```python
from build123d import *

# Parameters (mm, degrees)
SKETCH1_W           = 50
SKETCH1_H           = 100
BOSS_EXTRUDE1_DEPTH = 2.5
SKETCH2_R           = 1.25
BOSS_EXTRUDE2_DEPTH = 2.5
SKETCH4_W           = 15
SKETCH4_H           = 7.5
SKETCH4_H_2         = 33
CUT_EXTRUDE1_DEPTH  = 1


with BuildPart() as part:
    # Sketch1 → Boss-Extrude1 (new body, symmetric)
    with BuildSketch(Plane.XY):
        Rectangle(SKETCH1_W, SKETCH1_H)
    extrude(amount=BOSS_EXTRUDE1_DEPTH, both=True)

    # Sketch2 → Boss-Extrude2 (add)
    with BuildSketch(Plane.XY.offset(2.5)):
        with Locations((20, -10)):
            Circle(SKETCH2_R)
    boss_extrude2 = extrude(amount=BOSS_EXTRUDE2_DEPTH)

    # Sketch3 → Revolve1 (revolve)
    with BuildSketch(Plane(origin=(20, 0, 0), x_dir=(0, 0, -1), z_dir=(1, 0, 0))):
        with BuildLine():
            Line((-8, -6.75), (-8, -13.25))
            ThreePointArc((-8, -13.25), (-11.25, -10), (-8, -6.75))
        make_face()
    revolve1 = revolve(axis=Axis((20, -6.75, 8), (0, -1, 0)))

    # Sketch4 → Cut-Extrude1 (cut)
    with BuildSketch(Plane.XY.offset(2.5)):
        with Locations((-11.25, 37.25)):
            Rectangle(SKETCH4_W, SKETCH4_H)
        with Locations((11.25, 37.25)):
            Rectangle(SKETCH4_W, SKETCH4_H)
        with Locations((11.25, 10)):
            Rectangle(SKETCH4_W, SKETCH4_H_2)
        with Locations((-11.25, 10)):
            Rectangle(SKETCH4_W, SKETCH4_H_2)
        with Locations((-11.25, -30)):
            Rectangle(SKETCH4_W, SKETCH4_H_2)
        with Locations((11.25, -30)):
            Rectangle(SKETCH4_W, SKETCH4_H_2)
    cut_extrude1 = extrude(amount=-CUT_EXTRUDE1_DEPTH, mode=Mode.SUBTRACT)

    # Mirror1: Boss-Extrude2, Revolve1, Cut-Extrude1 across plane
    add(boss_extrude2.mirror(Plane.XY))
    add(revolve1.mirror(Plane.XY))
    add(cut_extrude1.mirror(Plane.XY), mode=Mode.SUBTRACT)


solid = part.part
```
Design review of the part built by this model. Coordinates are the model's own, in mm. A direction names the side the tool comes from. Round coordinates to 2 decimals unless told otherwise and drop trailing zeros. Write each loop counter-clockwise with the first axis right and the second up, starting at its lowest first coordinate (ties: lowest second). Pieces come first, ordered by that corner, then holes. Notation, with made-up numbers: (-14.75, -33) -> (24.25, -33) arc R31 ccw to (24.25, -2) -> close; hole circle Ø9 at (12, -40). An arc over 180 degrees is marked (long way). Write item = value, one per line. Start each with the question number.
1) Wall thickness on probe 1 along X at (y, z) = (-15, -1.75); probe 2 along Z at (x, y) = (10, -7); probe 3 along Z at (x, y) = (4, 37): over which ranges is each line inside the solid? List them lowest first. Write a range as from..to.
2) Mouldability with a two-part tool opening along X and no side actions: class faces 1 (the face through (-25, -1, 0)), 2 (the face through (11, 37, 1.5)), 3 (the face through (0, 1, 2.5)) as +X half, -X half, draft (parallel to the pull), parting line (faces both ways), or undercut.
3) Take a section at A-A, the plane y = -10. State the section outline as (x, z) points.
4) Take a section at B-B, the plane x = 12. State the section outline as (y, z) points.
5) Take a section at C-C, the plane x = 20. State the section outline as (y, z) points.
6) Take a section at D-D, the plane y = 44. State the section outline as (x, z) points.
7) Clearance check with flat-ended pins moving along their axes: pin 1 (12 mm diameter, centred on x = -15, y = 6, fed in from -Z); pin 2 (4 mm diameter, centred on x = 9, y = 36, fed in from -Z); pin 3 (7.5 mm diameter, centred on x = -11.5, y = 7, fed in from +Z). State where each tip first meets the part, or that it passes through.
8) Tool access review of faces 4 (the face through (0, 50, 0)), 5 (the face through (-11, 37, -1.5)), 6 (the face through (25, -1, 0)), 7 (the face through (-11, -30, 1.5)), 8 (the face through (21.19, -9.62, -3.73)): name each direction out of +Z, -Z, +X, -X, +Y, -Y from which nothing blocks a thin tool from reaching the whole face with its end or side.
Results list:
q1.probe_1 = -25..-18.75, -3.75..3.75, 18.75..25
q1.probe_2 = -2.5..2.5
q1.probe_3 = -1.5..1.5
q2.face_1 = -X half
q2.face_2 = undercut
q2.face_3 = draft
q3.outline = (-25, -2.5) -> (18.75, -2.5) -> (18.75, -5) arc R3.25 ccw (long way) to (21.25, -5) -> (21.25, -2.5) -> (25, -2.5) -> (25, 2.5) -> (21.25, 2.5) -> (21.25, 5) arc R3.25 ccw (long way) to (18.75, 5) -> (18.75, 2.5) -> (-25, 2.5) -> close
q4.outline = (-50, -2.5) -> (-46.5, -2.5) -> (-46.5, -1.5) -> (-13.5, -1.5) -> (-13.5, -2.5) -> (-6.5, -2.5) -> (-6.5, -1.5) -> (26.5, -1.5) -> (26.5, -2.5) -> (33.5, -2.5) -> (33.5, -1.5) -> (41, -1.5) -> (41, -2.5) -> (50, -2.5) -> (50, 2.5) -> (41, 2.5) -> (41, 1.5) -> (33.5, 1.5) -> (33.5, 2.5) -> (26.5, 2.5) -> (26.5, 1.5) -> (-6.5, 1.5) -> (-6.5, 2.5) -> (-13.5, 2.5) -> (-13.5, 1.5) -> (-46.5, 1.5) -> (-46.5, 2.5) -> (-50, 2.5) -> close
q5.outline = (-50, -2.5) -> (-11.25, -2.5) -> (-11.25, -5) arc R3.25 ccw (long way) to (-8.75, -5) -> (-8.75, -2.5) -> (50, -2.5) -> (50, 2.5) -> (-8.75, 2.5) -> (-8.75, 5) arc R3.25 ccw (long way) to (-11.25, 5) -> (-11.25, 2.5) -> (-50, 2.5) -> close
q6.outline = (-25, -2.5) -> (25, -2.5) -> (25, 2.5) -> (-25, 2.5) -> close
q7.pin_1 = -2.5
q7.pin_2 = -1.5
q7.pin_3 = 1.5
q8.face_4 = +Z, -Z, +X, -X, +Y
q8.face_5 = -Z
q8.face_6 = +Z, -Z, +X, +Y, -Y
q8.face_7 = +Z
q8.face_8 = none
